Verification items for the finished model (mm, model axes). A direction names the side the tool comes from. Give positions to 0.01 mm unless a question says otherwise; leave off trailing zeros. Loops run counter-clockwise (first coordinate to the right, second up) from the corner with the lowest first, then second, coordinate; pieces in that order, holes last. Notation, with made-up numbers: (81.25, -28.75) - (116.25, -28.75) arc R16 cw to (116.25, -0.75) - close; hole circle Ø3 at (70, 67). An arc over 180 degrees is marked (long way). One line per item, written item: value. Start each with the question number.
1. Sectioned sample at C-C (x = 2.75). Record the cut outline in (y, z).
2. Scan lines: L1, parallel to Z at x = 11.5, y = 0; L2, parallel to Z at x = 18, y = -3.75. Record each from-to range of solid material in increasing order. Write a range as [from, to].
3. Gauge pin test, flat ends, axial feed: pin 1 (7.5 mm diameter, centred on y = 0, z = 0, fed in from -X); pin 2 (1.5 mm diameter, centred on x = 18, z = -0.5, fed in from -Y); pin 3 (4 mm diameter, centred on x = 12.5, z = 3.5, fed in from -Y); pin 4 (2 mm diameter, centred on x = 4.5, z = 4.5, fed in from -Y). Record the tip position at first contact, or that the pin passes through.
4. Access from +Z, -Z, +X, -X, +Y, -Y to the whole of each face (thin tool, end or side, straight path). Record for faces 4 (the flat face through (0, 3, -2)), 5 (the cylindrical face through (11.59, -1.08, -4.88)).
5. Sectioned sample at A-A (z = 0). Record the cut outline in (x, y), plus the area to 3 significant figures.
6. Sectioned sample at D-D (y = 6). Record the cut outline in (x, z).
7. Mould release check, pull along Z, two halves, no side actions. Record for faces 1 (the cylindrical face through (0.86, -1.73, -7.81)), 2 (the flat face through (21.7, 2, 3)), 3 (the cylindrical face through (10.7, -2.23, 2.43)): pulls with the +Z half, pulls with the -Z half, needs draft (parallel to the pull), parting line crosses it, or undercut.
Autodesk Inventor part; units mm, degrees
ref_plane "Płaszczyzna początkowa" through (0, 0, 0) normal (1, 0, 0) x (0, 1, 0)
ref_plane "XZ Plane" through (0, 0, 0) normal (0, 1, 0) x (-1, 0, 0)
ref_plane "XY Plane" through (0, 0, 0) normal (0, 0, 1) x (1, 0, 0)
sketch "Szkic główny" plane through (0, 0, 0) normal (0, 0, 1) x (1, 0, 0)
  line L0 (0, 0) -> (21.7, 0)
  line L1 (0, 0) -> (0, 8)
  line L2 (1.7, 8) -> (1.7, 5)
  line L3 (0, 8) -> (1.7, 8)
  line L4 (21.7, 5) -> (21.7, 0)
  line L5 (1.7, 5) -> (21.7, 5)
  dimension "d3" = 16
  dimension "d4" = 10
revolve "Obrót1" add sketch "Szkic główny" angle 360 about axis through (0, 0, 0) along (1, 0, 0)
chamfer "Faza1" distance 0.5 angle 45 1 edges at (21.7, -5, 0) measured on face at (15.0333, 4.9353, -0.8021)
sketch "Szkic3" plane through (21.7, 0, 0) normal (1, 0, 0) x (0, 0, -1)
  point P0 (0, 0)
hole "Otwór1" at (21.7, 0, 0) direction (-1, 0, 0) diameter 6.6 depth 21.7
sketch "Szkic4" plane through (21.7, 0, 0) normal (1, 0, 0) x (0, 0, -1)
  point P0 (0, 0)
hole "Otwór2" at (21.7, 0, 0) direction (-1, 0, 0) diameter 6.6 depth 21.7
equation "\"Length\" = 21.7"
properties part number "Wał" material "Steel"
Results are:
1. outline: circle Ø10 at (0, 0); hole circle Ø6.6 at (0, 0)
2. L1: z = [-5, -3.3], [3.3, 5]
2. L2: z = [-3.31, 3.31]
3. pin 1: stops at x = 0
3. pin 2: stops at y = -5
3. pin 3: stops at y = -4.77
3. pin 4: stops at y = -3.57
4. face 4: +Z, -Z, -X, +Y, -Y
4. face 5: +X
5. outline: (0, -8) - (1.7, -8) - (1.7, -5) - (21.2, -5) - (21.7, -4.5) - (21.7, -3.3) - (0, -3.3) - close; (0, 3.3) - (21.7, 3.3) - (21.7, 4.5) - (21.2, 5) - (1.7, 5) - (1.7, 8) - (0, 8) - close
5. area: 83.7 mm^2
6. outline: (0, -5.29) - (1.7, -5.29) - (1.7, 5.29) - (0, 5.29) - close
7. face 1: parting line crosses it
7. face 2: needs draft
7. face 3: undercut
